```python
from build123d import *

# Parameters (mm, degrees)
ESQUISSE1_W             = 10
ESQUISSE1_H             = 20
BOSS_EXTRU_1_DEPTH      = 35
ESQUISSE2_W             = 7
ESQUISSE2_H             = 15
ENL_V_MAT_EXTRU_1_DEPTH = 30
ESQUISSE3_R             = 1.55
ENL_V_MAT_EXTRU_2_DEPTH = 38.416573868
ESQUISSE4_R             = 2.5
ENL_V_MAT_EXTRU_3_DEPTH = 5
ESQUISSE5_R             = 0.75
ENL_V_MAT_EXTRU_4_DEPTH = 2.5
CONG_1_R                = 2
ESQUISSE6_R             = 1.6
ENL_V_MAT_EXTRU_5_DEPTH = 42.533119315


with BuildPart() as part:
    # Esquisse1 → Boss.-Extru.1 (new body)
    with BuildSketch(Plane.XY):
        with Locations((5, 10)):
            Rectangle(ESQUISSE1_W, ESQUISSE1_H)
    extrude(amount=BOSS_EXTRU_1_DEPTH)

    # Esquisse2 → Enlèv. mat.-Extru.1 (cut)
    with BuildSketch(Plane.XY.offset(35)):
        with Locations((5, 10)):
            Rectangle(ESQUISSE2_W, ESQUISSE2_H)
    extrude(amount=-ENL_V_MAT_EXTRU_1_DEPTH, mode=Mode.SUBTRACT)

    # Esquisse3 → Enlèv. mat.-Extru.2 (cut, through all)
    with BuildSketch(Plane.XY.offset(5)):
        with Locations((5, 14.527380154)):
            Circle(ESQUISSE3_R)
        with Locations((5, 6.280248244)):
            Circle(ESQUISSE3_R)
    extrude(amount=-ENL_V_MAT_EXTRU_2_DEPTH, mode=Mode.SUBTRACT)

    # Esquisse4 → Enlèv. mat.-Extru.3 (cut)
    with BuildSketch(Plane(origin=(0, 20, 0), x_dir=(1, 0, 0), z_dir=(0, 1, 0))):
        with Locations(Location((4.86841115, -9.754551776, 0), (0, 0, 270))):
            Circle(ESQUISSE4_R)
    extrude(amount=-ENL_V_MAT_EXTRU_3_DEPTH, mode=Mode.SUBTRACT)

    # Esquisse5 → Enlèv. mat.-Extru.4 (cut)
    with BuildSketch(Plane.ZY):
        with Locations((30, 14)):
            Circle(ESQUISSE5_R)
        with Locations((30, 6)):
            Circle(ESQUISSE5_R)
    extrude(amount=-ENL_V_MAT_EXTRU_4_DEPTH, mode=Mode.SUBTRACT)

    # Congé1
    cong_1_edges = [part.edges().sort_by_distance(p)[0] for p in [
        (0, 20, 17.5),
        (10, 20, 17.5),
        (10, 0, 17.5),
        (0, 0, 17.5),
    ]]
    fillet(cong_1_edges, radius=CONG_1_R)

    # Esquisse6 → Enlèv. mat.-Extru.5 (cut, through all)
    with BuildSketch(Plane(origin=(10, 0, 0), x_dir=(0, 0, -1), z_dir=(1, 0, 0))):
        with Locations((-7, 5)):
            Circle(ESQUISSE6_R)
        with Locations((-18.24812381, 5)):
            Circle(ESQUISSE6_R)
    extrude(amount=-ENL_V_MAT_EXTRU_5_DEPTH, mode=Mode.SUBTRACT)


solid = part.part
```
The model under review builds one solid part; all positions refer to its coordinate system, in mm. A direction names the side the tool comes from. Round coordinates to 2 decimals unless told otherwise and drop trailing zeros. Order: outer loops, then holes, each group sorted by start corner. A loop starts at its lowest first (then second) coordinate and runs counter-clockwise, first axis right, second up. Notation, with made-up numbers: (-36.75, 12) -> (-31.75, 12) arc R15 cw to (-31.75, 20) -> close; hole circle Ø6 at (3, 60.5). An arc over 180 degrees is marked (long way). One line per item, written item: value. Start each with the question number.
Q1. Mouldability with a two-part tool opening along Y and no side actions: class faces 4 (the face through (0.57, 19.4, 17.74)), 5 (the face through (3.35, 18.77, 7.77)), 6 (the face through (5, 2.5, 20)) as released by +Y, released by -Y, zero draft, split by the parting line, or undercut.
Q2. Wall thickness on line 1 (Y direction, x = 5.5, z = 25); line 2 (X direction, y = 12.5, z = 20.5); line 3 (Y direction, x = 1.1, z = 30): over which ranges is each line inside the solid? List them lowest first.
Q3. Take a section at C-C (z = 14). Write out the cut boundary in (x, y), and give its area (3 significant figures).
Q4. Take a section at A-A (z = 30). Write out the cut boundary in (x, y), and give its area (3 significant figures).
Q5. Take a section at B-B (x = 4.25). Write out the cut boundary in (y, z), and give its area (3 significant figures).
Q6. Machinability: for faces 1 (the face through (9, 4, 17)), 2 (the face through (5, 17.5, 20)), 3 (the face through (0.74, 6.225, 30.715)), which of the approach directions +Z, -Z, +X, -X, +Y, -Y give a long, thin tool a straight path to every point of the face, cutting with its end or side? Answer none if there is none.
Q7. Clearance check with flat-ended pins moving along their axes: pin 1 Ø1.9 at (y, z) = (5, 18.25) entering from -X; pin 2 Ø1.5 at (x, z) = (3.5, 10.5) entering from +Y. State where each tip first meets the part, or that it passes through.
Q8. Take a section at D-D (y = 14). Write out the cut boundary in (x, z), and give its area (3 significant figures).
Reported:
1. face 4: released by +Y
1. face 5: zero draft
1. face 6: undercut
2. line 1: y = 0 to 2.5, 17.5 to 20
2. line 2: x = 0 to 1.5, 8.5 to 10
2. line 3: y = 0.21 to 5.25, 6.75 to 13.25, 14.75 to 19.79
3. outline: (0, 2) arc R2 ccw to (2, 0) -> (8, 0) arc R2 ccw to (10, 2) -> (10, 18) arc R2 ccw to (8, 20) -> (2, 20) arc R2 ccw to (0, 18) -> close; hole (1.5, 2.5) -> (8.5, 2.5) -> (8.5, 17.5) -> (1.5, 17.5) -> close
3. area: 91.6 mm2
4. outline: (0, 2) arc R2 ccw to (2, 0) -> (8, 0) arc R2 ccw to (10, 2) -> (10, 18) arc R2 ccw to (8, 20) -> (2, 20) arc R2 ccw to (0, 18) -> (0, 14.75) -> (1.5, 14.75) -> (1.5, 17.5) -> (8.5, 17.5) -> (8.5, 2.5) -> (1.5, 2.5) -> (1.5, 5.25) -> (0, 5.25) -> close; (0, 6.75) -> (1.5, 6.75) -> (1.5, 13.25) -> (0, 13.25) -> close
4. area: 87.1 mm2
5. outline: (0, 0) -> (4.92, 0) -> (4.92, 5) -> (2.5, 5) -> (2.5, 35) -> (0, 35) -> close; (7.64, 0) -> (13.17, 0) -> (13.17, 5) -> (7.64, 5) -> close; (15.88, 0) -> (20, 0) -> (20, 7.33) -> (17.5, 7.33) -> (17.5, 5) -> (15.88, 5) -> close; (17.5, 12.18) -> (20, 12.18) -> (20, 35) -> (17.5, 35) -> close
5. area: 211 mm2
6. face 1: +X, -X
6. face 2: +Z
6. face 3: -X
7. pin 1: passes through
7. pin 2: stops at y = 2.5
8. outline: (0, 0) -> (3.54, 0) -> (3.54, 5) -> (1.5, 5) -> (1.5, 29.25) -> (0, 29.25) -> close; (0, 30.75) -> (1.5, 30.75) -> (1.5, 35) -> (0, 35) -> close; (6.46, 0) -> (10, 0) -> (10, 35) -> (8.5, 35) -> (8.5, 5) -> (6.46, 5) -> close
8. area: 123 mm2
